Read the model definition and answer for the solid it produces. Units are mm, in the model's axes. Face numbers are marked on the shaded views. A direction names the side the tool comes from. Coordinates: 2 decimals unless noted, no trailing zeros. Write each loop counter-clockwise with the first axis right and the second up, starting at its lowest first coordinate (ties: lowest second). Pieces come first, ordered by that corner, then holes.
(1) The part is cut by section B-B, the plane y = 1.75. Determine the outline of the cut face in (x, z), and give its area (3 significant figures).
(2) Straight lines are drawn through the part: line 1 along X through (y, z) = (2.05, -28); line 2 along X through (y, z) = (1.85, -36); line 3 along Z through (x, y) = (-6, 0.25). For each, find the intervals that lie inside material, in ascending order.
(3) The part is cut by section C-C, the plane x = -7.25. Determine the outline of the cut face in (y, z).
(4) The part is cut by section A-A, the plane z = -28. Determine the outline of the cut face in (x, y), and give its area (3 significant figures).
(5) Determine the mould class of the marked faces 1, 2, 3 and 4 for opening direction Z: pulls with the +Z half, pulls with the -Z half, needs draft (parallel to the pull), parting line crosses it, or undercut.
(6) The part is cut by section D-D, the plane z = -36. Determine the outline of the cut face in (x, y), and give its area (3 significant figures).
(7) Which of the six approach directions +Z, -Z, +X, -X, +Y, -Y give full straight-line access (tool end or side, diameter ignored) to the marked faces 5 and 6?
(8) Given pin 1 (4 mm diameter, centred on x = -4.5, z = -32.5, fed in from -Y); pin 2 (5 mm diameter, centred on x = -3.5, z = -39.5, fed in from -Y); pin 3 (4 mm diameter, centred on x = 5, y = -3, fed in from +Z), each flat-ended and moving along its own axis, determine where each tip first touches the part or whether it passes through.
```python
from build123d import *

# Parameters (mm, degrees)
SKETCH_1_R               = 5
EXTRUDE_1_DEPTH          = 8
EXTRUDE_2_DEPTH          = 10
EXTRUDE_2_DEPTH_BACK     = 10
FILLET_1_R               = 0.5
SKETCH_6_R               = 1.6
SKETCH_6_R_2             = 1.1
CUT_EXTRUDE_1_DEPTH      = 67.938579217
CUT_EXTRUDE_2_DEPTH      = 67.199195672
CUT_EXTRUDE_2_DEPTH_BACK = 67.199195672
CUT_EXTRUDE_3_DEPTH      = 55.878761072
FILLET_2_R               = 1


with BuildPart() as part:
    # Sketch 1 → Extrude 1 (new body)
    with BuildSketch(Plane(origin=(0, 0, 0), x_dir=(1, 0, 0), z_dir=(0, 1, 0))):
        Polygon((11.547005384, 40), (-11.547005384, 40), (-40.414518843, -10), (-28.867513459, -30), (28.867513459, -30), (40.414518843, -10), align=None)
        with Locations(Location((0, 0, 0), (0, 0, 270))):
            Circle(SKETCH_1_R, mode=Mode.SUBTRACT)
    extrude(amount=EXTRUDE_1_DEPTH)

    # Sketch 2 → Extrude 2 (add, two sides: drawn at the far end of the back side and taken through both)
    with BuildSketch(Plane(origin=(0, 0, 0), x_dir=(0, 0, -1), z_dir=(1, 0, 0)).offset(-EXTRUDE_2_DEPTH_BACK)):
        Polygon((40, 8), (40, 0), (48.535898385, -4.92820323), (52, 1.07179677), align=None)
    extrude(amount=EXTRUDE_2_DEPTH + EXTRUDE_2_DEPTH_BACK)

    # Sketch 4 → Cut-Revolve 1 (revolve, cut)
    with BuildSketch(Plane(origin=(0, 0, 0), x_dir=(0, 0, -1), z_dir=(1, 0, 0))):
        with BuildLine():
            Line((50.219872981, 3.988526329), (45.119872981, -4.84493279))
            ThreePointArc((45.119872981, -4.84493279), (52.08660254, -2.97820323), (50.219872981, 3.988526329))
        make_face()
    revolve(axis=Axis((0, 2.57179677, -49.401923789), (0, -0.8660254037844388, 0.4999999999999997)), mode=Mode.SUBTRACT)

    # Fillet 1
    fillet_1_edges = [part.edges().sort_by_distance(p)[0] for p in [
        (-6.119151464, 1.07179677, -52),
        (-6.119151464, -4.92820323, -48.535898385),
        (6.119151464, -4.92820323, -48.535898385),
        (0, -1.556706503, -42.696294756),
        (6.119151464, 1.07179677, -52),
        (4.124318125, -1.92820323, -50.267949192),
        (0, 4.443293497, -46.160396371),
        (-4.124318125, -1.92820323, -50.267949192),
    ]]
    fillet(fillet_1_edges, radius=FILLET_1_R)

    # Sketch 6 → Cut-Extrude 1 (cut, through all)
    with BuildSketch(Plane(origin=(0, 8, 0), x_dir=(1, 0, 0), z_dir=(0, 1, 0))):
        with Locations(Location((-5, 36, 0), (0, 0, 270))):
            Circle(SKETCH_6_R)
        with Locations(Location((5, 36, 0), (0, 0, 270))):
            Circle(SKETCH_6_R)
        with Locations(Location((-5, 28, 0), (0, 0, 270))):
            Circle(SKETCH_6_R_2)
        with Locations(Location((5, 28, 0), (0, 0, 270))):
            Circle(SKETCH_6_R_2)
    extrude(amount=-CUT_EXTRUDE_1_DEPTH, mode=Mode.SUBTRACT)

    # Sketch 7 → Cut-Extrude 2 (cut, two sides: drawn at the far end of the back side and taken through both)
    with BuildSketch(Plane(origin=(0, 0, 0), x_dir=(0, 0, -1), z_dir=(1, 0, 0)).offset(-CUT_EXTRUDE_2_DEPTH_BACK)):
        Polygon((50.267949192, -1.92820323), (40, 4), (25, 4), (25, 0), (-30, 0), (-30, 8), (40, 8), (51.566987298, 1.32179677), (52, 1.07179677), (51.75, 0.638784068), align=None)
    extrude(amount=CUT_EXTRUDE_2_DEPTH + CUT_EXTRUDE_2_DEPTH_BACK, mode=Mode.SUBTRACT)

    # Sketch 8 → Cut-Extrude 3 (cut, through all)
    with BuildSketch(Plane(origin=(0, 4, 0), x_dir=(1, 0, 0), z_dir=(0, 1, 0))):
        Polygon((-10, 40), (-11.547005384, 40), (-20.207259422, 25), (-10, 25), align=None)
        Polygon((10, 40), (11.547005384, 40), (20.207259422, 25), (10, 25), align=None)
    extrude(amount=-CUT_EXTRUDE_3_DEPTH, mode=Mode.SUBTRACT)

    # Fillet 2
    fillet_2_edges = [part.edges().sort_by_distance(p)[0] for p in [
        (0, 0, -40),
    ]]
    fillet(fillet_2_edges, radius=FILLET_2_R)


solid = part.part
```
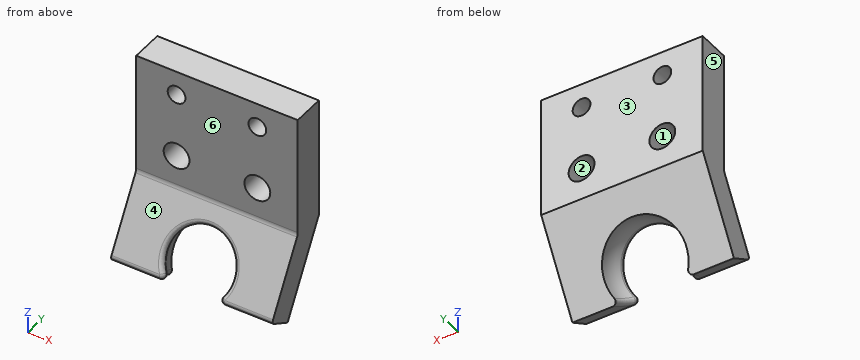
Computed:
1. outline: (-10, -43.9) - (-2.65, -43.9) arc R4.61 cw to (2.65, -43.9) - (10, -43.9) - (10, -25) - (-10, -25) - close; hole circle Ø3.2 at (-5, -36); hole circle Ø2.2 at (-5, -28); hole circle Ø3.2 at (5, -36); hole circle Ø2.2 at (5, -28)
1. area: 351 mm2
2. line 1: x = -10 to -6.1, -3.9 to 3.9, 6.1 to 10
2. line 2: x = -10 to -6.6, -3.4 to 3.4, 6.6 to 10
2. line 3: z = -46.5 to -37.25, -34.75 to -28.46, -27.54 to -25
3. outline: (-4.68, -48.1) arc R0.5 ccw to (-4.5, -48.79) - (-1.93, -50.27) - (4, -40) - (4, -25) - (0, -25) - (0, -39.73) arc R1 cw to (-0.13, -40.23) - close
4. outline: (-10, 0) - (-6.1, 0) - (-6.1, 4) - (-10, 4) - close; (-3.9, 0) - (3.9, 0) - (3.9, 4) - (-3.9, 4) - close; (6.1, 0) - (10, 0) - (10, 4) - (6.1, 4) - close
4. area: 62.4 mm2
5. face 1: undercut
5. face 2: undercut
5. face 3: needs draft
5. face 4: pulls with the +Z half
6. outline: (-10, 0) - (-6.6, 0) - (-6.6, 4) - (-10, 4) - close; (-3.4, 0) - (3.4, 0) - (3.4, 4) - (-3.4, 4) - close; (6.6, 0) - (10, 0) - (10, 4) - (6.6, 4) - close
6. area: 54.4 mm2
7. face 5: +Z, -Z, -X, +Y, -Y
7. face 6: +Z, +X, -X, -Y
8. pin 1: stops at y = 0
8. pin 2: stops at y = -1.15
8. pin 3: stops at z = -41.73
